from build123d import *


with BuildPart() as f1:
    # F0 (on Front) → F1 (revolve)
    with BuildSketch(Plane.XZ):
        Polygon((4.75, 0), (6.25, 0), (6.25, 5), (7, 10), (6.25, 10), (6.25, 30), (4.5, 34.808085), (4.5, 75), (3, 75), (3, 34.543595), (4.75, 29.73551), align=None)
    revolve(axis=Axis((0, 0, 35.781112), (0, 0, 1)))

    # F2 (on Right) → F3 (revolve)
    with BuildSketch(Plane.YZ):
        with BuildLine():
            Line((4.4, 65.285346), (4.4, 61.985346))
            ThreePointArc((4.4, 61.985346), (4.826595, 63.635346), (4.4, 65.285346))
        make_face()
    revolve(axis=Axis((0, 0, 60.848506), (0, 0, 1)))


solid = f1.part
The listing builds one solid part. Answer for the finished solid, in the listing's coordinates (mm). A direction names the side the tool comes from. Give positions to 0.01 mm unless a question says otherwise; leave off trailing zeros. Write each loop counter-clockwise with the first axis right and the second up, starting at its lowest first coordinate (ties: lowest second). Pieces come first, ordered by that corner, then holes.
Item 1: Find the intervals of material crossed by line 1 along Y through (x, z) = (0, 18.5); line 2 along Y through (x, z) = (0, 44); line 3 along X through (y, z) = (-0.25, 44.5), in increasing order.
Item 2: Section A-A, the plane z = 56.5 is taken. Write down the section's boundary in (x, y).
Item 3: Determine the mould class of faces 6 (the cylindrical face through (2.192, -4.214, 14.66)), 7 (the cylindrical face through (-0.59, 4.46, 48.69)), 8 (the flat face through (-3, 6, 10)) for opening direction X: released by +X, released by -X, zero draft, split by the parting line, or undercut.
Item 4: Section B-B, the plane z = 16.5 is taken. Write down the section's boundary in (x, y).
Item 5: Which of the six approach directions +Z, -Z, +X, -X, +Y, -Y give full straight-line access (tool end or side, diameter ignored) to faces 1 (the cylindrical face through (-3, 0, 54)), 2 (the conical face through (4.559, 1.436, 34.04)), 3 (the cylindrical face through (5.96, 1.88, 20.14)), 4 (the flat face through (1, -3, 75)), 5 (the cylindrical face through (5.96, 1.88, 2.54))?
Item 6: Flat-ended cylindrical pins translate along their axes: P1, Ø1, axis at y = -2, z = 63.5, coming from the +X side; P2, Ø1, axis at y = -2.5, z = 25, coming from the +X side; P3, Ø1, axis at x = 4.5, z = 10, coming from the -Y side. Find the tip coordinate at first contact, or state that the pin passes through.
Completed:
1. line 1: y = -6.25 to -4.75, 4.75 to 6.25
1. line 2: y = -4.5 to -3, 3 to 4.5
1. line 3: x = -4.49 to -2.99, 2.99 to 4.49
2. outline: circle Ø9 at (0, 0); hole circle Ø6 at (0, 0)
3. face 6: undercut
3. face 7: split by the parting line
3. face 8: zero draft
4. outline: circle Ø12.5 at (0, 0); hole circle Ø9.5 at (0, 0)
5. face 1: +Z, -Z
5. face 2: none
5. face 3: +Z
5. face 4: +Z, +X, -X, +Y, -Y
5. face 5: -Z
6. P1: stops at x = 4.59
6. P2: stops at x = 5.92
6. P3: stops at y = -5.74
